from build123d import *

# Parameters (mm, degrees)
SKETCH1_R               = 1
BOSS_EXTRUDE1_DEPTH     = 20
SKETCH2_R               = 0.95
BOSS_EXTRUDE2_DEPTH     = 2.5
CUT_EXTRUDE1_DEPTH      = 21.310096012
CUT_EXTRUDE1_DEPTH_BACK = 21.310096012
SKETCH3_W               = 6.5
SKETCH3_H               = 2.5
FILLET1_R               = 1
FILLET2_R               = 0.25


with BuildPart() as part:
    # Sketch1 → Boss-Extrude1 (new body)
    with BuildSketch(Plane(origin=(0, 0, 0), x_dir=(0, 0, -1), z_dir=(1, 0, 0))):
        Circle(SKETCH1_R)
    extrude(amount=BOSS_EXTRUDE1_DEPTH)

    # Sketch2 → Boss-Extrude2 (add, symmetric)
    with BuildSketch(Plane.XY):
        with BuildLine():
            Line((0, -2.125), (0, 2.125))
            Line((0, 2.125), (-5.06876613, 2.493422203))
            ThreePointArc((-5.06876613, 2.493422203), (-7.75, 0), (-5.06876613, -2.493422203))
            Line((-5.06876613, -2.493422203), (0, -2.125))
        make_face()
        with Locations((-5.25, 0)):
            Circle(SKETCH2_R, mode=Mode.SUBTRACT)
    extrude(amount=BOSS_EXTRUDE2_DEPTH, both=True)

    # Sketch3 → Cut-Extrude1 (cut, two sides: drawn at the far end of the back side and taken through both)
    with BuildSketch(Plane(origin=(0, 0, 0), x_dir=(1, 0, 0), z_dir=(0, 1, 0)).offset(-CUT_EXTRUDE1_DEPTH_BACK)):
        with Locations((-4.5, 0)):
            Rectangle(SKETCH3_W, SKETCH3_H)
    extrude(amount=CUT_EXTRUDE1_DEPTH + CUT_EXTRUDE1_DEPTH_BACK, mode=Mode.SUBTRACT)

    # Fillet1
    fillet1_edges = [part.edges().sort_by_distance(p)[0] for p in [
        (0, -2.125, 0),
        (0, 2.125, 0),
    ]]
    fillet(fillet1_edges, radius=FILLET1_R)

    # Fillet2
    fillet2_edges = [part.edges().sort_by_distance(p)[0] for p in [
        (-1.25, 2.215855988, 0),
        (-1.25, -2.215855988, 0),
        (-7.75, 0, -1.25),
        (-3.159383065, 2.354639096, -1.25),
        (-3.159383065, -2.354639096, -1.25),
        (-7.75, 0, 1.25),
        (-3.159383065, -2.354639096, 1.25),
        (-3.159383065, 2.354639096, 1.25),
        (-2.998136291, 2.342918908, 2.5),
        (-2.998136291, 2.342918908, -2.5),
        (-2.998136291, -2.342918908, 2.5),
        (0, 0, -2.5),
        (-0.267711277, -1.876041023, -2.5),
        (-0.267711277, 1.876041023, -2.5),
        (0, 0, 2.5),
        (-0.267711277, -1.876041023, 2.5),
        (-0.267711277, 1.876041023, 2.5),
        (-7.75, 0, 2.5),
        (-2.998136291, -2.342918908, -2.5),
        (-7.75, 0, -2.5),
    ]]
    fillet(fillet2_edges, radius=FILLET2_R)


solid = part.part
The model under review builds one solid part; all positions refer to its coordinate system, in mm. A direction names the side the tool comes from. Round coordinates to 2 decimals unless told otherwise and drop trailing zeros. Loops run counter-clockwise (first coordinate to the right, second up) from the corner with the lowest first, then second, coordinate; pieces in that order, holes last. Notation, with made-up numbers: (40.25, 23.5) -> (70.25, 23.5) arc R26 ccw to (70.25, 44.5) -> close; hole circle Ø9 at (70.5, 45.5). An arc over 180 degrees is marked (long way). Return JSON: item names as keys, results as strings.
(1) The part is to be moulded in two halves that separate along Y. For faces 1 (the cylindrical face through (-7.75, 0.06, 1.88)), 2 (the cylindrical face through (-4.37, -0.36, -1.88)), 3 (the flat face through (-1.25, 0, 0)), say which applies: released by +Y, released by -Y, zero draft, split by the parting line, or undercut.
Solved:
{"face 1": "split by the parting line", "face 2": "undercut", "face 3": "zero draft"}
(2) Add section D-D on x = 3.5. Write out the cut boundary in (y, z).
Solved:
{"outline": "circle Ø2 at (0, 0)"}
(3) For line 1 (X direction, y = 0, z = 1.95); line 2 (Y direction, x = -5.25, z = 1.9); line 3 (X direction, y = -1.2, z = 0.7), list the stretches that pass through material, from the lowest coordinate up.
Solved:
{"line 1": "-7.75 to -6.2, -4.3 to 0", "line 2": "-2.5 to -0.95, 0.95 to 2.5", "line 3": "-1.25 to 0"}
(4) For pin 1 (1.5 mm diameter, centred on x = 15.5, y = -1, fed in from +Z); pin 2 (0.8 mm diameter, centred on y = -0.5, z = 0.5, fed in from -X), all flat-tipped, find the tip position at first contact; note any pin that passes through.
Solved:
{"pin 1": "z = 0.97", "pin 2": "x = -1.25"}
(5) Add section A-A on z = 2. Write out the cut boundary in (x, y), plus the area to 3 significant figures.
Solved:
{"outline": "(-5.07, -2.49) -> (-0.93, -2.19) arc R1 ccw to (0, -1.2) -> (0, 1.2) arc R1 ccw to (-0.93, 2.19) -> (-5.07, 2.49) arc R2.5 ccw (long way) to start; hole circle Ø1.9 at (-5.25, 0)", "area": "30.9 mm2"}
(6) Add section C-C on z = 0.7. Write out the cut boundary in (x, y), plus the area to 3 significant figures.
Solved:
{"outline": "(-1.25, -1.95) arc R0.25 ccw to (-0.98, -2.2) -> (-0.93, -2.19) arc R1 ccw to (0, -1.2) -> (0, -0.71) -> (20, -0.71) -> (20, 0.71) -> (0, 0.71) -> (0, 1.2) arc R1 ccw to (-0.93, 2.19) -> (-0.98, 2.2) arc R0.25 ccw to (-1.25, 1.95) -> close", "area": "33.6 mm2"}
(7) For faces 4 (the flat face through (-2.988, 2.342, 1.677)), 5 (the flat face through (-4, 0, 1.25)), 6 (the cylindrical face through (10, -1, 0)), list the 3-axis set-ups (+Z, -Z, +X, -X, +Y, -Y) from which the entire face can be reached by the end or side of a thin tool; tool diameter is ignored.
Solved:
{"face 4": "+Z, -Z, +X, +Y", "face 5": "-X, +Y, -Y", "face 6": "+X"}
(8) Add section B-B on y = 0. Write out the cut boundary in (x, z), plus the area to 3 significant figures.
Solved:
{"outline": "(-7.75, -2.25) arc R0.25 ccw to (-7.5, -2.5) -> (-6.2, -2.5) -> (-6.2, -1.25) -> (-7.5, -1.25) arc R0.25 ccw to (-7.75, -1.5) -> close; (-7.75, 1.5) arc R0.25 ccw to (-7.5, 1.25) -> (-6.2, 1.25) -> (-6.2, 2.5) -> (-7.5, 2.5) arc R0.25 ccw to (-7.75, 2.25) -> close; (-4.3, -2.5) -> (-0.25, -2.5) arc R0.25 ccw to (0, -2.25) -> (0, -1) -> (20, -1) -> (20, 1) -> (0, 1) -> (0, 2.25) arc R0.25 ccw to (-0.25, 2.5) -> (-4.3, 2.5) -> (-4.3, 1.25) -> (-1.25, 1.25) -> (-1.25, -1.25) -> (-4.3, -1.25) -> close", "area": "57.7 mm2"}
